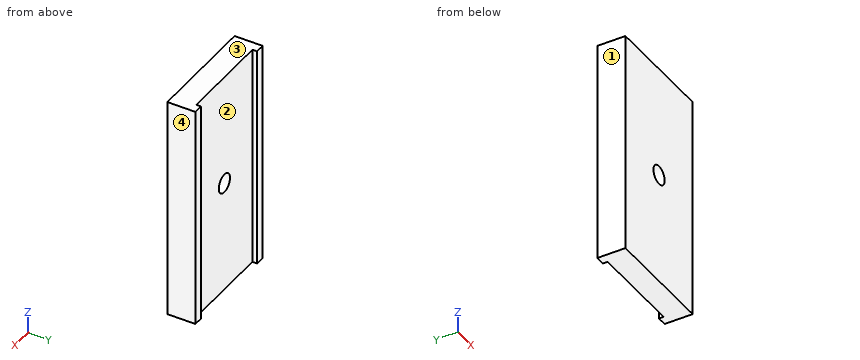
Autodesk Inventor part; units mm, degrees
ref_plane "YZ Plane" through (0, 0, 0) normal (1, 0, 0) x (0, 1, 0)
ref_plane "XZ Plane" through (0, 0, 0) normal (0, 1, 0) x (-1, 0, 0)
ref_plane "XY Plane" through (0, 0, 0) normal (0, 0, 1) x (1, 0, 0)
sketch "Sketch1" plane through (0, 0, 0) normal (0, 1, 0) x (-1, 0, 0)
  line L0 (0, 0) -> (-24, 0)
  line L1 (-24, 0) -> (-24, -48)
  line L2 (-24, -48) -> (0, -48)
  line L3 (0, -48) -> (0, 0)
  circle A0 centre (-12, -24) radius 2
  point P0 (-24, -24)
  point P1 (-12, 0)
  dimension "d0" = 24
  dimension "d1" = 48
  dimension "d2" = 4
extrude "Extrusion1" add sketch "Sketch1" along normal blind 6
sketch "Sketch2" plane through (0, 6, 0) normal (0, 1, 0) x (1, 0, 0)
  line L0 (2, 75.3172) -> (22, 75.3172)
  line L1 (22, 75.3172) -> (22, -3.0502)
  line L2 (22, -3.0502) -> (2, -3.0502)
  line L3 (2, -3.0502) -> (2, 75.3172)
  line L4 (0, 48) -> (0, 0)
  dimension "d5" = 20
  dimension "d6" = 2
extrude "Extrusion2" cut sketch "Sketch2" against normal blind 1
properties part number "centershortNEW"
Read the model definition and answer for the solid it produces. Units are mm, in the model's axes. Face numbers are marked on the shaded views. Coordinates: 2 decimals unless noted, no trailing zeros. Write each loop counter-clockwise with the first axis right and the second up, starting at its lowest first coordinate (ties: lowest second). Pieces come first, ordered by that corner, then holes. Notation, with made-up numbers: (4.5, 24.5) -> (17.5, 24.5) arc R15 ccw to (17.5, 41.5) -> close; hole circle Ø7 at (6, 47.5). An arc over 180 degrees is marked (long way). Return JSON: item names as keys, results as strings.
(1) The part is cut by section C-C on z = -39.5. Give the vertices of the cut face in (x, y).
Answers below:
{"outline": "(0, 0) -> (24, 0) -> (24, 6) -> (22, 6) -> (22, 5) -> (2, 5) -> (2, 6) -> (0, 6) -> close"}
(2) Each of these flat-tipped pins is pushed along its axis until it touches: P1, Ø1, axis at x = 6, z = -16, coming from the -Y side; P2, Ø6, axis at x = 18, z = -7, coming from the +Y side. Where does it stop, or does it pass through?
Answers below:
{"P1": "y = 0", "P2": "y = 5"}
(3) The part is cut by section D-D on x = 21.5. Give the vertices of the cut face in (y, z), then the cut area to 3 significant figures.
Answers below:
{"outline": "(0, -48) -> (5, -48) -> (5, 0) -> (0, 0) -> close", "area": "240 mm^2"}
(4) The part is cut by section B-B on z = -24. Give the vertices of the cut face in (x, y).
Answers below:
{"outline": "(0, 0) -> (10, 0) -> (10, 5) -> (2, 5) -> (2, 6) -> (0, 6) -> close; (14, 0) -> (24, 0) -> (24, 6) -> (22, 6) -> (22, 5) -> (14, 5) -> close"}
(5) Consider line 1 along X through (y, z) = (1.6, -24); line 2 along Z through (x, y) = (12, 3.75); line 3 along X through (y, z) = (5.45, -26.5). Determine where each line is inside the solid, lowest interval first. Write a range as from..to.
Answers below:
{"line 1": "0..10, 14..24", "line 2": "-48..-26, -22..0", "line 3": "0..2, 22..24"}
(6) The part is cut by section A-A on x = 12. Give the vertices of the cut face in (y, z), then the cut area to 3 significant figures.
Answers below:
{"outline": "(0, -48) -> (5, -48) -> (5, -26) -> (0, -26) -> close; (0, -22) -> (5, -22) -> (5, 0) -> (0, 0) -> close", "area": "220 mm^2"}
(7) For a pull along X with two mould halves and no side action, classify the marked faces 1, 2, 3 and 4 as pulls with the +X half, pulls with the -X half, needs draft (parallel to the pull), parting line crosses it, or undercut.
Answers below:
{"face 1": "pulls with the -X half", "face 2": "undercut", "face 3": "needs draft", "face 4": "pulls with the +X half"}
